Could you check a few things on this model? Use its own coordinates, in mm. Coordinates: 2 decimals unless noted, no trailing zeros. Order: outer loops, then holes, each group sorted by start corner. A loop starts at its lowest first (then second) coordinate and runs counter-clockwise, first axis right, second up. Notation, with made-up numbers: (-18, -20.5) -> (1, -20.5) arc R7 ccw to (1, -7.5) -> close; hole circle Ø6 at (57.5, 38.5). An arc over 180 degrees is marked (long way). Use a Markdown table: item, result. Add a question column.
1) Will this pin go through, and if not, where does the flat tip stop? pin 1 Ø4 at (x, z) = (-143, -37) entering from +Y.
2) If we section it at A-A (z = 0): Write out the boundary of the cut face in (x, y) (3 decimals), plus the area to 3 significant figures.
3) If we section it at B-B (x = 0): Write out the boundary of the cut face in (y, z) (3 decimals).
4) If we section it at D-D (x = 139): Write out the boundary of the cut face in (y, z) (3 decimals), plus the area to 3 significant figures.
5) If I drill on L1, parallel to X at y = 0.3, z = 0 (3 decimals); L2, parallel to X at y = 0.55, z = 0 (3 decimals); L3, parallel to Z at x = -201, y = -0.1, over which ranges is the centre line in solid material (lowest first)? Write a range as [from, to].
6) If we section it at C-C (y = -0.2): Write out the boundary of the cut face in (x, z) (3 decimals).
```python
from build123d import *

# Parameters (mm, degrees)
SKETCH1_W           = 342.9
SKETCH1_H           = 342.9
BOSS_EXTRUDE1_DEPTH = 0.4064
SKETCH4_W           = 342.9
SKETCH4_H           = 0.8128
BOSS_EXTRUDE3_DEPTH = 92.075
CIRPATTERN1_COUNT   = 4
FILLET1_R           = 19.05
SKETCH7_R           = 85.725
CUT_EXTRUDE1_DEPTH  = 88.9
SKETCH7_3_R         = 86.58225
SKETCH7_3_R_2       = 85.725
BOSS_EXTRUDE4_DEPTH = 0.2032


with BuildPart() as part:
    # Sketch1 → Boss-Extrude1 (new, symmetric)
    with BuildSketch(Plane(origin=(0, 0, 0), x_dir=(1, 0, 0), z_dir=(0, 1, 0))):
        Rectangle(SKETCH1_W, SKETCH1_H)
    extrude(amount=BOSS_EXTRUDE1_DEPTH, both=True)

    # Sketch4 → Boss-Extrude3 (add)
    with BuildSketch(Plane.ZY.offset(171.45)):
        Rectangle(SKETCH4_W, SKETCH4_H)
    boss_extrude3 = extrude(amount=BOSS_EXTRUDE3_DEPTH)

    # CirPattern1: Boss-Extrude3 ×4 about axis
    cirpattern1_axis = Axis((0, 0, 0), (0, 1, 0))
    for i in range(1, CIRPATTERN1_COUNT):
        add(boss_extrude3.rotate(cirpattern1_axis, i * 360 / CIRPATTERN1_COUNT))

    # Fillet1
    fillet1_edges = [part.edges().sort_by_distance(p)[0] for p in [
        (-171.45, 0, -171.45),
        (171.45, 0, -171.45),
        (-171.45, 0, 171.45),
        (171.45, 0, 171.45),
    ]]
    fillet(fillet1_edges, radius=FILLET1_R)

    # Sketch7 → Cut-Extrude1 (cut)
    with BuildSketch(Plane(origin=(0, 0.4064, 0), x_dir=(1, 0, 0), z_dir=(0, 1, 0))):
        with Locations(Location((0, 0, 0), (0, 0, 270))):
            Circle(SKETCH7_R)
    extrude(amount=-CUT_EXTRUDE1_DEPTH, mode=Mode.SUBTRACT)

    # Sketch7_3 → Boss-Extrude4 (add, symmetric)
    with BuildSketch(Plane(origin=(0, 0.4064, 0), x_dir=(1, 0, 0), z_dir=(0, 1, 0))):
        with Locations(Location((0, 0, 0), (0, 0, 90))):
            Circle(SKETCH7_3_R)
        with Locations(Location((0, 0, 0), (0, 0, 270))):
            Circle(SKETCH7_3_R_2, mode=Mode.SUBTRACT)
    extrude(amount=BOSS_EXTRUDE4_DEPTH, both=True)


solid = part.part
```
Answer sheet:
| question | item | result |
|---|---|---|
| 1 | pin 1 | y = 0.41 |
| 2 | outline | (-263.525, -0.406) -> (-85.725, -0.406) -> (-85.725, 0.61) -> (-86.582, 0.61) -> (-86.582, 0.406) -> (-263.525, 0.406) -> close; (85.725, -0.406) -> (263.525, -0.406) -> (263.525, 0.406) -> (86.582, 0.406) -> (86.582, 0.61) -> (85.725, 0.61) -> close |
| 2 | area | 289 mm2 |
| 3 | outline | (-0.406, -263.525) -> (0.406, -263.525) -> (0.406, -86.582) -> (0.61, -86.582) -> (0.61, -85.725) -> (-0.406, -85.725) -> close; (-0.406, 85.725) -> (0.61, 85.725) -> (0.61, 86.582) -> (0.406, 86.582) -> (0.406, 263.525) -> (-0.406, 263.525) -> close |
| 4 | outline | (-0.406, -263.525) -> (0.406, -263.525) -> (0.406, 263.525) -> (-0.406, 263.525) -> close |
| 4 | area | 428 mm2 |
| 5 | L1 | [-263.525, -85.725], [85.725, 263.525] |
| 5 | L2 | [-86.582, -85.725], [85.725, 86.582] |
| 5 | L3 | [-171.45, 171.45] |
| 6 | outline | (-263.525, -171.45) -> (-190.5, -171.45) arc R19.05 cw to (-171.45, -190.5) -> (-171.45, -263.525) -> (171.45, -263.525) -> (171.45, -190.5) arc R19.05 cw to (190.5, -171.45) -> (263.525, -171.45) -> (263.525, 171.45) -> (190.5, 171.45) arc R19.05 cw to (171.45, 190.5) -> (171.45, 263.525) -> (-171.45, 263.525) -> (-171.45, 190.5) arc R19.05 cw to (-190.5, 171.45) -> (-263.525, 171.45) -> close; hole circle Ø171.45 at (0, 0) |
